Read the model definition and answer for the solid it produces. Units are mm, in the model's axes. Face numbers are marked on the shaded views. Coordinates: 2 decimals unless noted, no trailing zeros. Loops run counter-clockwise (first coordinate to the right, second up) from the corner with the lowest first, then second, coordinate; pieces in that order, holes last. Notation, with made-up numbers: (48, 38.25) - (58, 38.25) arc R34 ccw to (58, 74.25) - close; hole circle Ø2 at (3, -28.75). An arc over 180 degrees is marked (long way). One line per question, with ' | ' between items. Start each with the question number.
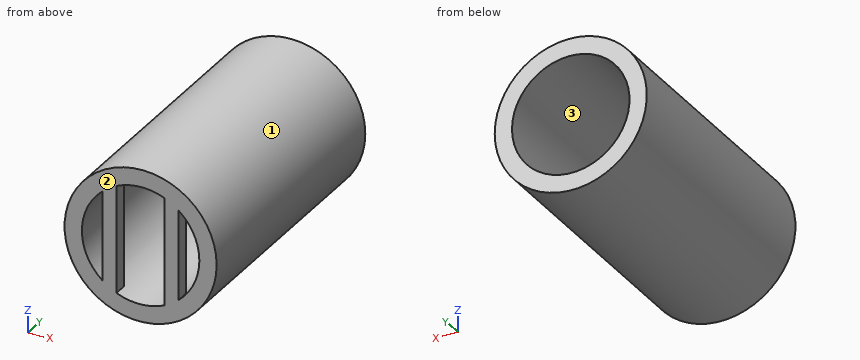
```python
from build123d import *

# Parameters (mm, degrees)
F0_R     = 13.97
F1_DEPTH = 50.8
F2_R     = 10.795
F3_DEPTH = 50.8
F5_DEPTH = 2.54


with BuildPart() as f1:
    # F0 (on Front) → F1 (new body)
    with BuildSketch(Plane.XZ):
        Circle(F0_R)
    extrude(amount=F1_DEPTH)

    # F2 (on face) → F3 (cut)
    with BuildSketch(Plane.XZ.offset(50.8)):
        Circle(F2_R)
    extrude(amount=-F3_DEPTH, mode=Mode.SUBTRACT)

    # F4 (on face) → F5 (join)
    with BuildSketch(Plane.XZ.offset(50.8)):
        with BuildLine():
            ThreePointArc((-6.973512343, -8.2402761242), (-5.7595656887, -9.1301384479), (-4.4336462139, -9.8425))
            Line((-4.4336462139, -9.8425), (-4.4336462139, 9.8425))
            ThreePointArc((-4.4336462139, 9.8425), (-5.7595656887, 9.1301384479), (-6.973512343, 8.2402761242))
            Line((-6.973512343, 8.2402761242), (-6.973512343, -8.2402761242))
        make_face()
    extrude(amount=-F5_DEPTH)

    # F6: F1 across plane


with BuildPart() as f1_1:
    add(f1.part)
    add(f1.part.mirror(Plane.YZ))


solid = f1_1.part
```
1) The part is cut by section A-A on x = 0. Write down the section's boundary in (y, z) (3 decimals).
2) The part is cut by section B-B on z = 0. Write down the section's boundary in (x, y) (3 decimals), and give its area (3 significant figures).
3) The mould has two halves that part along X. Classify the marked faces 1, 2 and 3: released by +X, released by -X, zero draft, split by the parting line, or undercut.
4) The part is cut by section D-D on z = -7.5. Write down the section's boundary in (x, y).
5) Given pin 1 Ø1 at (x, z) = (8, -3) entering from -Y; pin 2 Ø2 at (x, z) = (5.5, 3.5) entering from +Y; pin 3 Ø1.5 at (y, z) = (-43.5, -2) entering from +X; pin 4 Ø3 at (x, y) = (-11, -21) entering from +Z, each flat-ended and moving along its own axis, determine where each tip first touches the part or whether it passes through.
6) Find the intervals of material crossed by line 1 along X through (y, z) = (-33.5, 0) (3 decimals); line 2 along X through (y, z) = (-34, 1), in increasing order. Write a range as from..to.
7) The part is cut by section C-C on y = -24. Write down the section's boundary in (x, z) (3 decimals).
Answer below:
1) outline: (-50.8, -13.97) - (0, -13.97) - (0, -10.795) - (-50.8, -10.795) - close; (-50.8, 10.795) - (0, 10.795) - (0, 13.97) - (-50.8, 13.97) - close
2) outline: (-13.97, -50.8) - (-10.795, -50.8) - (-10.795, 0) - (-13.97, 0) - close; (-6.974, -50.8) - (-4.434, -50.8) - (-4.434, -48.26) - (-6.974, -48.26) - close; (4.434, -50.8) - (6.974, -50.8) - (6.974, -48.26) - (4.434, -48.26) - close; (10.795, -50.8) - (13.97, -50.8) - (13.97, 0) - (10.795, 0) - close | area: 335 mm2
3) face 1: split by the parting line | face 2: zero draft | face 3: undercut
4) outline: (-11.79, -50.8) - (-7.76, -50.8) - (-7.76, 0) - (-11.79, 0) - close; (-6.97, -50.8) - (-4.43, -50.8) - (-4.43, -48.26) - (-6.97, -48.26) - close; (4.43, -50.8) - (6.97, -50.8) - (6.97, -48.26) - (4.43, -48.26) - close; (7.76, -50.8) - (11.79, -50.8) - (11.79, 0) - (7.76, 0) - close
5) pin 1: through | pin 2: y = -48.26 | pin 3: x = 13.91 | pin 4: z = 10.24
6) line 1: -13.97..-10.795, 10.795..13.97 | line 2: -13.93..-10.75, 10.75..13.93
7) outline: circle Ø27.94 at (0, 0); hole circle Ø21.59 at (0, 0)
